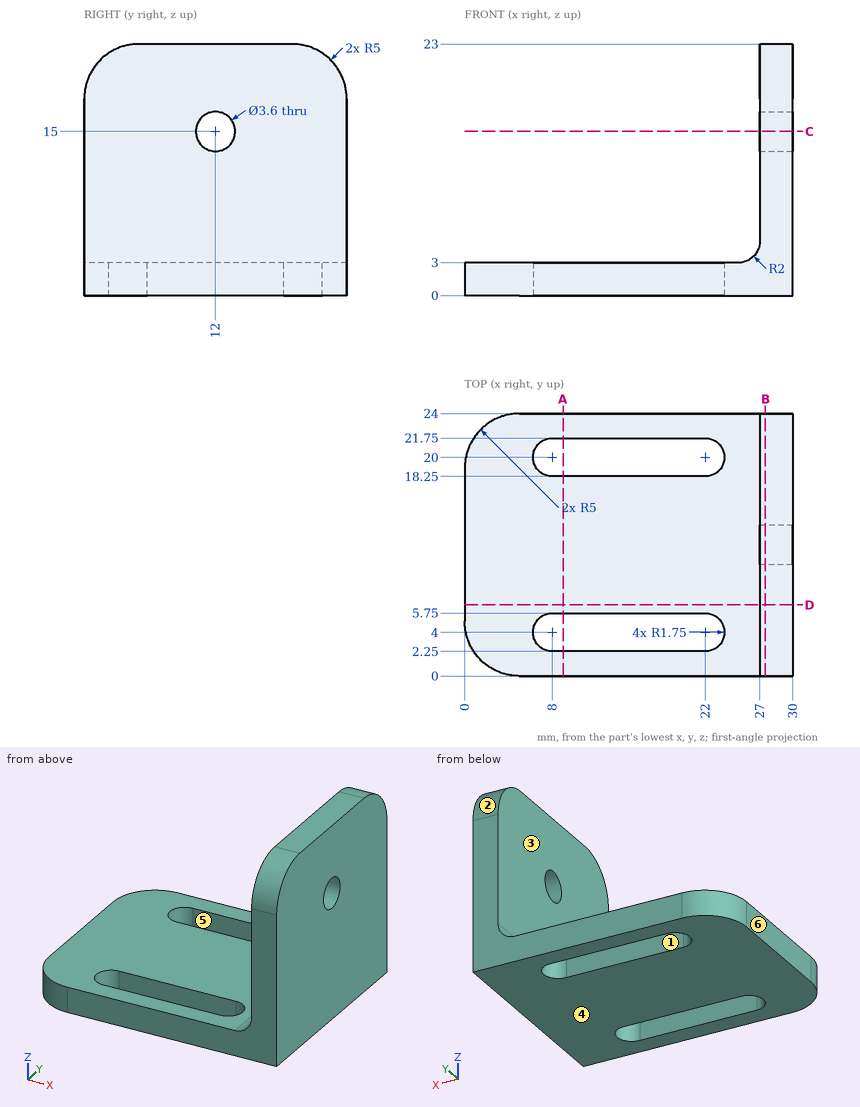
Can you work these out from the drawing? Everything is in mm from the part's minimum corner. A direction names the side the tool comes from. Coordinates: 2 decimals unless noted, no trailing zeros. Order: outer loops, then holes, each group sorted by start corner. A loop starts at its lowest first (then second) coordinate and runs counter-clockwise, first axis right, second up. Notation, with made-up numbers: (-31, -38) -> (-22, -38) arc R26 ccw to (-22, -20) -> close; hole circle Ø4 at (2.25, -19). An arc over 180 degrees is marked (long way). Return JSON: item names as keys, results as strings.
1) On a 3-axis mill with a long thin cutter (end or side, diameter ignored), from which of +Z, -Z, +X, -X, +Y, -Y can I reach the whole of each face in a straight line? I mean the marked faces 1, 2 and 3. Say none if no direction works.
Conclusion:
{"face 1": "+Z, -Z", "face 2": "+Z, +X, -X, +Y", "face 3": "+Z, -X, +Y, -Y"}
2) If we section it at C-C on z = 15: List the corners of the cut face in (x, y) for me, plus the area to 3 significant figures.
Conclusion:
{"outline": "(27, 0) -> (30, 0) -> (30, 10.2) -> (27, 10.2) -> close; (27, 13.8) -> (30, 13.8) -> (30, 24) -> (27, 24) -> close", "area": "61.2 mm²"}
3) If I drill on probe 1 along Z at (x, y) = (27.85, 12); probe 2 along Z at (x, y) = (22.75, 17.25); probe 3 along X at (y, z) = (10, 19.5), over which ranges is the centre line in solid material (lowest first)?
Conclusion:
{"probe 1": "z = 0 to 13.2, 16.8 to 23", "probe 2": "z = 0 to 3", "probe 3": "x = 27 to 30"}
4) If we section it at B-B on x = 27.5: List the corners of the cut face in (y, z) for me, plus the area to 3 significant figures.
Conclusion:
{"outline": "(0, 0) -> (24, 0) -> (24, 18) arc R5 ccw to (19, 23) -> (5, 23) arc R5 ccw to (0, 18) -> close; hole circle Ø3.6 at (12, 15)", "area": "531 mm²"}
5) If we section it at D-D on y = 6.5: List the corners of the cut face in (x, z) for me, plus the area to 3 significant figures.
Conclusion:
{"outline": "(0, 0) -> (30, 0) -> (30, 23) -> (27, 23) -> (27, 5) arc R2 cw to (25, 3) -> (0, 3) -> close", "area": "151 mm²"}
6) Thinking about a two-plate mould opening in X: for the marked faces 4, 5 and 6, which applies, +X half, -X half, draft (parallel to the pull), parting line (faces both ways), or undercut?
Conclusion:
{"face 4": "draft", "face 5": "undercut", "face 6": "-X half"}
7) If we section it at A-A on x = 9: List the corners of the cut face in (y, z) for me.
Conclusion:
{"outline": "(0, 0) -> (2.25, 0) -> (2.25, 3) -> (0, 3) -> close; (5.75, 0) -> (18.25, 0) -> (18.25, 3) -> (5.75, 3) -> close; (21.75, 0) -> (24, 0) -> (24, 3) -> (21.75, 3) -> close"}
8) I'm going to push flat-ended pins straight in: P1, Ø1.5, axis at x = 6.5, y = 15, coming from the +Z side; P2, Ø4.5, axis at y = 12, z = 15, coming from the -X side; P3, Ø0.9, axis at x = 17.5, z = 2, coming from the -Y side. Where does each tip first touch, or does it pass through?
Conclusion:
{"P1": "stops at z = 3", "P2": "stops at x = 27", "P3": "stops at y = 0"}
